Can you work these out from the model? Positions are in its coordinate system, mm. Face numbers are marked on the shaded views. Round coordinates to 2 decimals unless told otherwise and drop trailing zeros. Loops run counter-clockwise (first coordinate to the right, second up) from the corner with the lowest first, then second, coordinate; pieces in that order, holes last. Notation, with made-up numbers: (-12.5, 87.5) -> (41.5, 87.5) arc R33 ccw to (41.5, 121.5) -> close; hole circle Ø7 at (53.5, 6). An arc over 180 degrees is marked (long way). Write item = value, one per line.
from build123d import *

# Parameters (mm, degrees)
M3X0_5_TAPPED_HOLE1_D           = 2.5
M3X0_5_TAPPED_HOLE1_CSINK_D     = 3.05
M3X0_5_TAPPED_HOLE1_CSINK_ANGLE = 90


with BuildPart() as part:
    # Sketch1 → Revolve1 (revolve)
    with BuildSketch(Plane.XY, mode=Mode.PRIVATE) as revolve1_sk:
        Polygon((4, 0), (4, 10), (11, 10), (11, 6), (6, 6), (6, 0), align=None)
    revolve(revolve1_sk.sketch.rotate(Axis((0, 0, 0), (0, 1, 0)), 90), axis=Axis((0, 0, 0), (0, 1, 0)))

    # M3x0.5 Tapped Hole1 (through all)
    with Locations(Plane(origin=(0, 10, 0), x_dir=(1, 0, 0), z_dir=(0, 1, 0))):
        with Locations((0, 8), (8, 0), (0, -8), (-8, 0), (0, 0)):
            CounterSinkHole(M3X0_5_TAPPED_HOLE1_D / 2, M3X0_5_TAPPED_HOLE1_CSINK_D / 2, counter_sink_angle=M3X0_5_TAPPED_HOLE1_CSINK_ANGLE)


solid = part.part
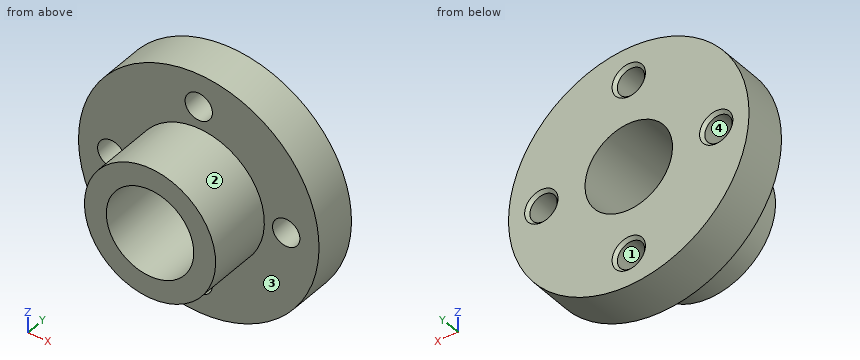
1. Suppose I cut it at D-D, the plane y = 4.25. List the corners of the cut face in (x, z) for me, and give its area (3 significant figures).
Entries:
outline = circle Ø12 at (0, 0); hole circle Ø8 at (0, 0)
area = 62.8 mm²
2. Suppose I cut it at B-B, the plane x = 8. List the corners of the cut face in (y, z) for me (3 decimals), and give its area (3 significant figures).
Entries:
outline = (6, -7.55) -> (10, -7.55) -> (10, -1.525) -> (9.725, -1.25) -> (6, -1.25) -> close; (6, 1.25) -> (9.725, 1.25) -> (10, 1.525) -> (10, 7.55) -> (6, 7.55) -> close
area = 50.3 mm²
3. We'd pull the mould along Z, two halves only. Please class the marked faces 1, 2, 3 and 4: released by +Z, released by -Z, zero draft, split by the parting line, or undercut.
Entries:
face_1 = undercut
face_2 = split by the parting line
face_3 = zero draft
face_4 = undercut
4. Suppose I cut it at C-C, the plane z = -8. List the corners of the cut face in (x, y) for me (3 decimals).
Entries:
outline = (-7.55, 6) -> (-1.25, 6) -> (-1.25, 9.725) -> (-1.525, 10) -> (-7.55, 10) -> close; (1.25, 6) -> (7.55, 6) -> (7.55, 10) -> (1.525, 10) -> (1.25, 9.725) -> close
5. Suppose I cut it at A-A, the plane z = 0. List the corners of the cut face in (x, y) for me (3 decimals).
Entries:
outline = (-11, 6) -> (-9.25, 6) -> (-9.25, 9.725) -> (-9.525, 10) -> (-11, 10) -> close; (-6.75, 6) -> (-6, 6) -> (-6, 0) -> (-4, 0) -> (-4, 10) -> (-6.475, 10) -> (-6.75, 9.725) -> close; (4, 0) -> (6, 0) -> (6, 6) -> (6.75, 6) -> (6.75, 9.725) -> (6.475, 10) -> (4, 10) -> close; (9.25, 6) -> (11, 6) -> (11, 10) -> (9.525, 10) -> (9.25, 9.725) -> close
6. I'm going to push flat-ended pins straight in: pin 1 (2 mm diameter, centred on x = -8, y = 8, fed in from -Z); pin 2 (4 mm diameter, centred on y = 8.5, z = -6, fed in from -X); pin 3 (5 mm diameter, centred on x = -4, z = -8, fed in from -Y). Where does each tip first touch, or does it pass through?
Entries:
pin_1 = -8.49
pin_2 = -10.25
pin_3 = 6
7. I need wall thicknesses on line 1 (Y direction, x = 7.5, z = 2.5); line 2 (X direction, y = 7.85, z = 8). Which ranges of each line are inside material? Lowest first, please. Write a range as [from, to].
Entries:
line_1 = [6, 10]
line_2 = [-7.55, -1.25], [1.25, 7.55]
